from build123d import *

# Parameters (mm, degrees)
SKETCH002_AS_DRAWN_R                      = 1.6
EXTRUDE001_DEPTH                          = 4.5
EXTRUDE001_ONTO_SKETCH002_ROLL_ANGLE      = 90
EXTRUDE001_ONTO_SKETCH002_PLACEMENT_ANGLE = 180
EXTRUDE_DEPTH                             = 3
SKETCH001_R                               = 12.063289
PAD_DEPTH                                 = 3
SKETCH003_R                               = 8
POCKET_DEPTH                              = 3.001
FILLET_R                                  = 0.9


with BuildPart() as extrude001:
    # Sketch002 as drawn → Extrude001 (new)
    with BuildSketch(Plane.XY):
        with BuildLine():
            Line((-8.765843, 14.9), (-21.5, 14.9))
            Line((-21.5, 14.9), (-21.5, 3))
            Line((-21.5, 3), (21.5, 3))
            Line((21.5, 3), (21.5, 14.9))
            Line((21.5, 14.9), (8.765843, 14.9))
            ThreePointArc((-8.765843, 14.9), (0, 11.5), (8.765843, 14.9))
        make_face()
        with Locations((-15.55, 8.95)):
            Circle(SKETCH002_AS_DRAWN_R, mode=Mode.SUBTRACT)
        with Locations((15.55, 8.95)):
            Circle(SKETCH002_AS_DRAWN_R, mode=Mode.SUBTRACT)
    extrude(amount=-EXTRUDE001_DEPTH)


with BuildPart() as extrude001_1:
    # Extrude001 onto Sketch002 roll: moved
    add(extrude001.part.rotate(Axis((0, 0, 0), (1, 0, 0)), EXTRUDE001_ONTO_SKETCH002_ROLL_ANGLE))


with BuildPart() as extrude001_2:
    # Extrude001 onto Sketch002 placement: moved
    add(extrude001_1.part.moved(Location((0, 83.136711, 0))).rotate(Axis((0, 83.136711, 0), (0, 0, 1)), EXTRUDE001_ONTO_SKETCH002_PLACEMENT_ANGLE))


with BuildPart() as fillet_body:
    # Sketch → Extrude (new body)
    with BuildSketch(Plane.XY):
        with BuildLine():
            Line((-21.5, 83.136711), (21.5, 83.136711))
            Line((21.5, 83.136711), (21.5, 73.136711))
            ThreePointArc((17.748453, 62.850809), (20.531425, 67.662881), (21.5, 73.136711))
            ThreePointArc((17.748453, 62.850809), (5.730319, 35.123847), (10.819042, 5.335848))
            ThreePointArc((-10.819042, 5.335848), (0, -12.063289), (10.819042, 5.335848))
            ThreePointArc((-10.819042, 5.335848), (-5.733751, 35.124931), (-17.75562, 62.850809))
            ThreePointArc((-21.5, 73.136711), (-20.534792, 67.663591), (-17.75562, 62.850809))
            Line((-21.5, 83.136711), (-21.5, 73.136711))
        make_face()
    extrude(amount=EXTRUDE_DEPTH)

    # Sketch001 → Pad (new body)
    with BuildSketch(Plane.XY.offset(3)):
        Circle(SKETCH001_R)
        Polygon((0, 7.563289), (-6.55, 3.781644), (-6.55, -3.781644), (0, -7.563289), (6.55, -3.781644), (6.55, 3.781644), align=None, mode=Mode.SUBTRACT)
    extrude(amount=PAD_DEPTH)

    # Fusion: union Extrude001
    add(extrude001_2.part)

    # Sketch003 → Pocket (cut, through all)
    with BuildSketch(Plane.XY.offset(3)):
        with Locations((-0.002934, 63.657442)):
            Circle(SKETCH003_R)
    extrude(amount=-POCKET_DEPTH, mode=Mode.SUBTRACT)

    # Fillet
    fillet_edges = [fillet_body.edges().sort_by_distance(p)[0] for p in [
        (-21.5, 78.136711, 0),
        (0, 83.136711, 0),
        (-20.534792, 67.663591, 0),
        (21.5, 78.136711, 0),
        (-5.733751, 35.124931, 0),
        (20.531425, 67.662881, 0),
        (0, -12.063289, 0),
        (5.730319, 35.123847, 0),
        (-8.002934, 63.657442, 0),
    ]]
    fillet(fillet_edges, radius=FILLET_R)


solid = fillet_body.part
CAD build for the part. Positions are in the model's coordinates, mm. A direction names the side the tool comes from. Round coordinates to 2 decimals unless told otherwise and drop trailing zeros. Loops run counter-clockwise (first coordinate to the right, second up) from the corner with the lowest first, then second, coordinate; pieces in that order, holes last.
(1) Cut at B-B (z = 13). Give the cut face in (x, y).
(2) Cut at A-A (z = 4). Give the cut face in (x, y).
(3) Two-plate mould, pull along Y, no slides. Class faces 4 (the cylindrical face through (5.783, 35.55, 1.935)), 5 (the cylindrical face through (-14.28, 80.92, 7.98)), 6 (the cylindrical face through (20.504, 67.589, 1.935)), 7 (the cylindrical face through (-1.74, 55.85, 1.96)): +Y half, -Y half, draft (parallel to the pull), parting line (faces both ways), or undercut.
(4) Wall check: line 1 along Z through (x, y) = (15.55, 79.8); line 2 along Y through (x, z) = (1, 4.5); line 3 along Y through (x, z) = (-15.5, 12). Give the ranges that are in metal, low to high.
(5) Drop flat-ended pins along their axis: pin 1 (14.5 mm diameter, centred on x = 0, y = -0.5, fed in from +Z); pin 2 (4 mm diameter, centred on y = 36, z = 3.5, fed in from -X); pin 3 (3.5 mm diameter, centred on x = 15.55, z = 8.95, fed in from -Y). Give the stop position or say it passes through.
(6) Which spindle directions (+Z, -Z, +X, -X, +Y, -Y) get a long thin tool onto all of the face, cutting with end or side? Do faces 1 (the flat face through (-6.55, 0, 4)), 2 (the flat face through (5, -5, 6)), 3 (the cylindrical face through (-5.684, 34.699, 1.935)). Say none if no direction does.
Findings below:
1. outline: (-21.5, 78.64) - (-6.06, 78.64) - (-6.06, 83.14) - (-21.5, 83.14) - close; (6.06, 78.64) - (21.5, 78.64) - (21.5, 83.14) - (6.06, 83.14) - close
2. outline: (-21.5, 78.64) - (21.5, 78.64) - (21.5, 83.14) - (-21.5, 83.14) - close; circle Ø24.13 at (0, 0); hole (-6.55, -3.78) - (0, -7.56) - (6.55, -3.78) - (6.55, 3.78) - (0, 7.56) - (-6.55, 3.78) - close
3. face 4: undercut
3. face 5: draft
3. face 6: -Y half
3. face 7: undercut
4. line 1: z = 0 to 7.35, 10.55 to 14.9
4. line 2: y = -12.02 to -6.99, 6.99 to 12.02, 78.64 to 83.14
4. line 3: y = 78.64 to 83.14
5. pin 1: stops at z = 6
5. pin 2: stops at x = -6.15
5. pin 3: stops at y = 78.64
6. face 1: +Z
6. face 2: +Z, +X, -X, -Y
6. face 3: +Z, -Z, -X
